Autodesk Inventor part; units mm, degrees
ref_plane "YZ Plane" through (0, 0, 0) normal (1, 0, 0) x (0, 1, 0)
ref_plane "XZ Plane" through (0, 0, 0) normal (0, 1, 0) x (-1, 0, 0)
ref_plane "XY Plane" through (0, 0, 0) normal (0, 0, 1) x (1, 0, 0)
sketch "Sketch1" plane through (0, 0, 0) normal (0, 0, 1) x (1, 0, 0)
  line L0 (0, 0) -> (152.4, 0)
  line L1 (152.4, 0) -> (152.4, -101.6)
  line L2 (152.4, -101.6) -> (0, -101.6)
  line L3 (0, -101.6) -> (0, 0)
  dimension "d0" = 152.4
  dimension "d1" = 101.6
extrude "Extrusion1" add sketch "Sketch1" along normal blind 12.7
sketch "Sketch2" plane through (0, 0, 12.7) normal (0, 0, 1) x (1, 0, 0)
  circle A0 centre (12.7, -12.7) radius 3.81
  line L0 (0, 0) -> (0, -101.6)
  line L1 (152.4, 0) -> (0, 0)
  dimension "d4" = 7.62
  dimension "d5" = 12.7
  dimension "d6" = 12.7
extrude "Extrusion2" add sketch "Sketch2" along normal blind 12.7
pattern_linear "Rectangular Pattern1" count 4 spacing 25.4 along (0, -1, 0) count 6 spacing 25.4 along (1, 0, 0) of "Extrusion2"
properties part number "AWRectangular Pattern5.5a"
Could you check a few things on this model? Use its own coordinates, in mm. A direction names the side the tool comes from. Give positions to 0.01 mm unless a question says otherwise; leave off trailing zeros. Write each loop counter-clockwise with the first axis right and the second up, starting at its lowest first coordinate (ties: lowest second). Pieces come first, ordered by that corner, then holes. Notation, with made-up numbers: (67.25, 79.5) - (126.25, 79.5) arc R28 ccw to (126.25, 103.5) - close; hole circle Ø6 at (13.5, -0.75). An arc over 180 degrees is marked (long way). One line per item, written item: value. Start each with the question number.
Item 1: Imagine slicing it at D-D, the plane y = -81.5. List the corners of the cut face in (x, z) for me.
Item 2: I'm going to push flat-ended pins straight in: pin 1 (10 mm diameter, centred on x = 113.5, y = -28, fed in from +Z); pin 2 (4 mm diameter, centred on y = -86, z = 18.5, fed in from +X); pin 3 (3 mm diameter, centred on y = -61, z = 14, fed in from +X). Where does each tip first touch, or does it pass through?
Item 3: Which directions (+Z, -Z, +X, -X, +Y, -Y) give clear straight access to the entire face, cutting with the end or side of a thin tool? Please do faces 4 (the face through (62.67, -59.78, 18.96)), 5 (the face through (63, -38, 25.4)).
Item 4: Please list where these lines run through material, in increasing order: line 1 (Y direction, x = 64, z = 14.25); line 2 (Y direction, x = 91.5, z = 15.75); line 3 (Z direction, x = 33.5, y = -96.5). Write a range as from..to.
Item 5: Imagine slicing it at C-C, the plane y = -12.7. List the corners of the cut face in (x, z) for me.
Item 6: Imagine slicing it at B-B, the plane z = 20.25. Give the number of separate pieces and of enclosed holes in the cut face, and give its area (3 significant figures).
Item 7: If we mould it in two halves opening along Y, with no side actions, what happens to faces 1 (the face through (75, 0, 6)), 2 (the face through (89, -89, 25.4)), 3 (the face through (11.87, -34.38, 18.96))? For each: +Y half, -Y half, draft (parallel to the pull), parting line (faces both ways), or undercut.
Item 8: Imagine slicing it at A-A, the plane x = 139.7. List the corners of the cut face in (y, z) for me, and give its area (3 significant figures).
Geometry says:
1. outline: (0, 0) - (152.4, 0) - (152.4, 12.7) - (0, 12.7) - close
2. pin 1: z = 12.7
2. pin 2: x = 143.4
2. pin 3: x = 152.4
3. face 4: +Z
3. face 5: +Z, +X, -X, +Y, -Y
4. line 1: -92.68..-85.12, -67.28..-59.72, -41.88..-34.32, -16.48..-8.92
4. line 2: -91.68..-86.12, -66.28..-60.72, -40.88..-35.32, -15.48..-9.92
4. line 3: 0..12.7
5. outline: (0, 0) - (152.4, 0) - (152.4, 12.7) - (143.51, 12.7) - (143.51, 25.4) - (135.89, 25.4) - (135.89, 12.7) - (118.11, 12.7) - (118.11, 25.4) - (110.49, 25.4) - (110.49, 12.7) - (92.71, 12.7) - (92.71, 25.4) - (85.09, 25.4) - (85.09, 12.7) - (67.31, 12.7) - (67.31, 25.4) - (59.69, 25.4) - (59.69, 12.7) - (41.91, 12.7) - (41.91, 25.4) - (34.29, 25.4) - (34.29, 12.7) - (16.51, 12.7) - (16.51, 25.4) - (8.89, 25.4) - (8.89, 12.7) - (0, 12.7) - close
6. separate pieces: 24
6. enclosed holes: 0
6. area: 1,090 mm^2
7. face 1: +Y half
7. face 2: draft
7. face 3: undercut
8. outline: (-101.6, 0) - (0, 0) - (0, 12.7) - (-8.89, 12.7) - (-8.89, 25.4) - (-16.51, 25.4) - (-16.51, 12.7) - (-34.29, 12.7) - (-34.29, 25.4) - (-41.91, 25.4) - (-41.91, 12.7) - (-59.69, 12.7) - (-59.69, 25.4) - (-67.31, 25.4) - (-67.31, 12.7) - (-85.09, 12.7) - (-85.09, 25.4) - (-92.71, 25.4) - (-92.71, 12.7) - (-101.6, 12.7) - close
8. area: 1,680 mm^2
